```python
from build123d import *

# Parameters (mm, degrees)
SKETCH1_W           = 203.2
SKETCH1_H           = 101.6
BOSS_EXTRUDE1_DEPTH = 6.35
SKETCH2_W           = 6.35
SKETCH2_H           = 12.7
CUT_EXTRUDE1_DEPTH  = 6.35
SKETCH5_W           = 6.35
SKETCH5_H           = 6.35
CUT_EXTRUDE2_DEPTH  = 6.35
LPATTERN1_COUNT     = 15
LPATTERN1_PITCH     = 12.7
SKETCH6_W           = 6.35
SKETCH6_H           = 6.35
CUT_EXTRUDE3_DEPTH  = 6.35
LPATTERN2_COUNT     = 7
LPATTERN2_PITCH     = 12.7
CUT_EXTRUDE4_DEPTH  = 6.35
SKETCH8_W           = 6.35
SKETCH8_H           = 6.35
CUT_EXTRUDE5_DEPTH  = 6.35
SKETCH10_W          = 6.35
SKETCH10_H          = 6.35
CUT_EXTRUDE6_DEPTH  = 6.35
LPATTERN3_COUNT     = 3
LPATTERN3_PITCH     = 12.7


with BuildPart() as part:
    # Sketch1 → Boss-Extrude1 (new body)
    with BuildSketch(Plane(origin=(0, 0, 0), x_dir=(0, 0, -1), z_dir=(1, 0, 0))):
        with Locations((101.6, 50.8)):
            Rectangle(SKETCH1_W, SKETCH1_H)
    extrude(amount=-BOSS_EXTRUDE1_DEPTH)

    # Sketch2 → Cut-Extrude1 (cut)
    with BuildSketch(Plane.XZ):
        with Locations((-3.175, -196.85)):
            Rectangle(SKETCH2_W, SKETCH2_H)
    extrude(amount=-CUT_EXTRUDE1_DEPTH, mode=Mode.SUBTRACT)

    # Sketch5 → Cut-Extrude2 (cut)
    with BuildSketch(Plane.XZ):
        with Locations((-3.175, -180.975)):
            Rectangle(SKETCH5_W, SKETCH5_H)
    cut_extrude2 = extrude(amount=-CUT_EXTRUDE2_DEPTH, mode=Mode.SUBTRACT)

    # LPattern1: Cut-Extrude2 ×15
    with Locations(*[(0, 0, i * LPATTERN1_PITCH) for i in range(1, LPATTERN1_COUNT)]):
        add(cut_extrude2, mode=Mode.SUBTRACT)

    # Sketch6 → Cut-Extrude3 (cut)
    with BuildSketch(Plane(origin=(0, 0, -203.2), x_dir=(-1, 0, 0), z_dir=(0, 0, -1))):
        with Locations((3.175, 15.875)):
            Rectangle(SKETCH6_W, SKETCH6_H)
    cut_extrude3 = extrude(amount=-CUT_EXTRUDE3_DEPTH, mode=Mode.SUBTRACT)

    # LPattern2: Cut-Extrude3 ×7
    with Locations(*[(0, i * LPATTERN2_PITCH, 0) for i in range(1, LPATTERN2_COUNT)]):
        add(cut_extrude3, mode=Mode.SUBTRACT)

    # Sketch7 → Cut-Extrude4 (cut)
    with BuildSketch(Plane(origin=(0, 0, 0), x_dir=(0, 0, -1), z_dir=(1, 0, 0))):
        Polygon((0, 101.6), (0, 50.8), (50.8, 101.6), align=None)
    extrude(amount=-CUT_EXTRUDE4_DEPTH, mode=Mode.SUBTRACT)

    # Sketch8 → Cut-Extrude5 (cut)
    with BuildSketch(Plane.XY):
        with Locations((-3.175, 9.525)):
            Rectangle(SKETCH8_W, SKETCH8_H)
    extrude(amount=-CUT_EXTRUDE5_DEPTH, mode=Mode.SUBTRACT)

    # Sketch10 → Cut-Extrude6 (cut)
    with BuildSketch(Plane.XY):
        with Locations((-3.175, 22.225)):
            Rectangle(SKETCH10_W, SKETCH10_H)
    cut_extrude6 = extrude(amount=-CUT_EXTRUDE6_DEPTH, mode=Mode.SUBTRACT)

    # LPattern3: Cut-Extrude6 ×3
    with Locations(*[(0, i * LPATTERN3_PITCH, 0) for i in range(1, LPATTERN3_COUNT)]):
        add(cut_extrude6, mode=Mode.SUBTRACT)


solid = part.part
```
Check sheet for the modelled part. Datum: model origin and axes. Units: mm. A direction names the side the tool comes from. Give positions to 0.01 mm unless a question says otherwise; leave off trailing zeros. Loops run counter-clockwise (first coordinate to the right, second up) from the corner with the lowest first, then second, coordinate; pieces in that order, holes last. Notation, with made-up numbers: (80, -35) - (138, -35) arc R21 cw to (138, -8) - close; hole circle Ø8 at (-32.5, -7.5). An arc over 180 degrees is marked (long way). One line per question, with ' | ' between items. Start each with the question number.
1. Cross-section at B-B, the plane y = 67. Enter the section's corners in (x, z), plus the area to 3 significant figures.
2. Material ranges on line 1 along Y through (x, z) = (-5.25, -154.5); line 2 along Z through (x, y) = (-1, 14); line 3 along Z through (x, y) = (-0.75, 33.5), recorded low to high. Write a range as [from, to].
3. Gauge pin test, flat ends, axial feed: pin 1 Ø3 at (x, z) = (-2.5, -4.5) entering from -Y; pin 2 Ø3 at (x, z) = (-2.5, -198.5) entering from -Y; pin 3 Ø3 at (x, y) = (-4, 37) entering from +Z; pin 4 Ø1.9 at (x, y) = (-3, 3) entering from +Z. Record the tip position at first contact, or that the pin passes through.
4. Set-up check for faces 4 (the flat face through (-3, 0, -86)), 5 (the flat face through (-3, 6.35, -197)), 6 (the flat face through (-3, 3, -158.75)), 7 (the flat face through (-3, 63.5, -200)): record each of +Z, -Z, +X, -X, +Y, -Y from which the full face is reachable in a straight line by a thin tool's end or side.
5. Draft check along Z on faces 1 (the flat face through (-3, 0, -9)), 2 (the flat face through (-3, 3, -190.5)), 3 (the flat face through (-3, 6.35, -29)). Enter one of: released by +Z, released by -Z, zero draft, split by the parting line, or undercut.
6. Cross-section at A-A, the plane z = -142. Enter the section's corners in (x, y).
Check result:
1) outline: (-6.35, -196.85) - (0, -196.85) - (0, -16.2) - (-6.35, -16.2) - close | area: 1,150 mm2
2) line 1: y = [6.35, 101.6] | line 2: z = [-196.85, 0] | line 3: z = [-203.2, -6.35]
3) pin 1: stops at y = 12.7 | pin 2: stops at y = 6.35 | pin 3: stops at z = 0 | pin 4: stops at z = -6.35
4) face 4: +Z, -Z, +X, -X, -Y | face 5: -Z, +X, -X, -Y | face 6: +X, -X, -Y | face 7: -Z, +X, -X
5) face 1: zero draft | face 2: released by -Z | face 3: undercut
6) outline: (-6.35, 6.35) - (0, 6.35) - (0, 101.6) - (-6.35, 101.6) - close
